Source: CAD feature listing. Evaluate the final solid. Frame: model axes, mm. A direction names the side the tool comes from. Round coordinates to 2 decimals unless told otherwise and drop trailing zeros. Order: outer loops, then holes, each group sorted by start corner. A loop starts at its lowest first (then second) coordinate and runs counter-clockwise, first axis right, second up. Notation, with made-up numbers: (86.25, 54) - (118.25, 54) arc R20 cw to (118.25, 67) - close; hole circle Ø8 at (-2, 81.25). An arc over 180 degrees is marked (long way). Put each result on its own line as item: value. Start each with the question number.
1) Section A-A on y = 0. Output: boundary loops of the cut face in (x, z).
2) Line query: probe 1 along Y at (x, z) = (100, 17.5); probe 2 along Z at (x, y) = (64, 1.5); probe 3 along Z at (x, y) = (102, 19). Output: solid intervals per line, ascending. Write a range as [from, to].
3) Access query for faces 5 (the face through (-4.336, -19.524, 24.93)), 6 (the face through (51, -30, 10)). Directions: +Z, -Z, +X, -X, +Y, -Y. A direction counts if a zero-diameter tool reaches every point of the face in a straight line with its end or side. Return the directions, or none.
4) Contact query for flat-ended pins moving along their axis: P1, Ø2, axis at y = -6, z = 10, coming from the -X side; P2, Ø2, axis at x = 102, y = 19.5, coming from the +Z side; P3, Ø1, axis at x = 101, z = 10.5, coming from the +Y side. Output: stop coordinate, or through.
5) Section D-D on x = 110. Output: boundary loops of the cut face in (y, z), then the cut area to 3 significant figures.
6) Section B-B on x = 89. Output: boundary loops of the cut face in (y, z).
7) Mould query, pull axis X, two halves, no side actions, for faces 1 (the face through (49, 30, 10)), 2 (the face through (100, 0, 10)), 3 (the face through (80.02, 0.88, 15.07)), 4 (the face through (129.993, 0.66, 9.86)). Classes: +X half, -X half, draft (parallel to the pull), parting line (faces both ways), or undercut.
8) Section C-C on z = 3.5. Output: boundary loops of the cut face in (x, y).
```python
from build123d import *

# Parameters (mm, degrees)
SALIENTE_EXTRUIR1_DEPTH = 20
CROQUIS2_R              = 20
SALIENTE_EXTRUIR2_DEPTH = 10
CROQUIS3_R              = 20
CORTAR_EXTRUIR1_DEPTH   = 10


with BuildPart() as part:
    # Croquis1 → Saliente-Extruir1 (new body)
    with BuildSketch(Plane.XY):
        with BuildLine():
            Line((0, 30), (100, 30))
            ThreePointArc((100, 30), (130, 0), (100, -30))
            Line((100, -30), (0, -30))
            ThreePointArc((0, -30), (-30, 0), (0, 30))
        make_face()
    extrude(amount=SALIENTE_EXTRUIR1_DEPTH)

    # Croquis2 → Saliente-Extruir2 (add)
    with BuildSketch(Plane.XY.offset(20)):
        Circle(CROQUIS2_R)
    extrude(amount=SALIENTE_EXTRUIR2_DEPTH)

    # Croquis3 → Cortar-Extruir1 (cut)
    with BuildSketch(Plane.XY.offset(20)):
        with Locations((100, 0)):
            Circle(CROQUIS3_R)
    extrude(amount=-CORTAR_EXTRUIR1_DEPTH, mode=Mode.SUBTRACT)


solid = part.part
```
Answer sheet:
1. outline: (-30, 0) - (130, 0) - (130, 20) - (120, 20) - (120, 10) - (80, 10) - (80, 20) - (20, 20) - (20, 30) - (-20, 30) - (-20, 20) - (-30, 20) - close
2. probe 1: [-30, -20], [20, 30]
2. probe 2: [0, 20]
2. probe 3: [0, 10]
3. face 5: +Z
3. face 6: +Z, -Z, +X, -X, -Y
4. P1: x = -29.58
4. P2: z = 20
4. P3: y = 30
5. outline: (-28.28, 0) - (28.28, 0) - (28.28, 20) - (17.32, 20) - (17.32, 10) - (-17.32, 10) - (-17.32, 20) - (-28.28, 20) - close
5. area: 785 mm^2
6. outline: (-30, 0) - (30, 0) - (30, 20) - (16.7, 20) - (16.7, 10) - (-16.7, 10) - (-16.7, 20) - (-30, 20) - close
7. face 1: draft
7. face 2: undercut
7. face 3: undercut
7. face 4: +X half
8. outline: (0, -30) - (100, -30) arc R30 ccw to (100, 30) - (0, 30) arc R30 ccw to start
